Geometry check sheet. Reference: the model listing, model coordinates, mm. A direction names the side the tool comes from. Coordinates: 2 decimals unless noted, no trailing zeros. Loops run counter-clockwise (first coordinate to the right, second up) from the corner with the lowest first, then second, coordinate; pieces in that order, holes last.
from build123d import *

# Parameters (mm, degrees)
F0_W     = 80
F0_H     = 60
F1_DEPTH = 40
F2_W     = 20
F2_H     = 60
F3_DEPTH = 20
F4_W     = 60
F4_H     = 60
F5_DEPTH = 10


with BuildPart() as f1:
    # F0 (on Front) → F1 (new body)
    with BuildSketch(Plane.XZ):
        with Locations((40, 30)):
            Rectangle(F0_W, F0_H)
    extrude(amount=F1_DEPTH)

    # F2 (on face) → F3 (cut)
    with BuildSketch(Plane.XZ.offset(40)):
        with Locations((10, 30)):
            Rectangle(F2_W, F2_H)
        with Locations((70, 30)):
            Rectangle(F2_W, F2_H)
    extrude(amount=-F3_DEPTH, mode=Mode.SUBTRACT)

    # F4 (on face) → F5 (cut)
    with BuildSketch(Plane(origin=(0, 0, 0), x_dir=(-1, 0, 0), z_dir=(0, 1, 0))):
        with Locations((-40, 30)):
            Rectangle(F4_W, F4_H)
    extrude(amount=-F5_DEPTH, mode=Mode.SUBTRACT)


solid = f1.part
(1) Gauge pin test, flat ends, axial feed: pin 1 Ø22 at (x, z) = (74.5, 32) entering from -Y; pin 2 Ø22 at (y, z) = (-33.5, 33) entering from +X; pin 3 Ø1 at (x, z) = (20.5, 33) entering from +Y. Record the tip position at first contact, or that the pin passes through.
Findings:
pin 1: stops at y = -20
pin 2: stops at x = 60
pin 3: stops at y = -10
(2) Sectioned sample at D-D on y = -30. Record the cut outline in (x, z), and give its area (3 significant figures).
Findings:
outline: (20, 0) - (60, 0) - (60, 60) - (20, 60) - close
area: 2,400 mm2
(3) Scan lines: L1, parallel to X at y = -3, z = 54.5; L2, parallel to X at y = -28, z = 14; L3, parallel to Y at x = 22, z = 41.5. Record each from-to range of solid material in increasing order.
Findings:
L1: x = 0 to 10, 70 to 80
L2: x = 20 to 60
L3: y = -40 to -10
(4) Sectioned sample at B-B on z = 40. Record the cut outline in (x, y), and give its area (3 significant figures).
Findings:
outline: (0, -20) - (20, -20) - (20, -40) - (60, -40) - (60, -20) - (80, -20) - (80, 0) - (70, 0) - (70, -10) - (10, -10) - (10, 0) - (0, 0) - close
area: 1,800 mm2
(5) Sectioned sample at C-C on x = 14.5. Record the cut outline in (y, z).
Findings:
outline: (-20, 0) - (-10, 0) - (-10, 60) - (-20, 60) - close
(6) Access from +Z, -Z, +X, -X, +Y, -Y to the whole of each face (thin tool, end or side, straight path). Record for faces 5 (the flat face through (10, -20, 30)), 6 (the flat face through (70, -20, 30)), 7 (the flat face through (70, -5, 30)).
Findings:
face 5: +Z, -Z, -X, -Y
face 6: +Z, -Z, +X, -Y
face 7: +Z, -Z, +Y
(7) Sectioned sample at A-A on y = -7.5. Record the cut outline in (x, z).
Findings:
outline: (0, 0) - (10, 0) - (10, 60) - (0, 60) - close; (70, 0) - (80, 0) - (80, 60) - (70, 60) - close
(8) Draft check along X on faces 1 (the flat face through (20, -30, 30)), 2 (the flat face through (5, 0, 30)), 3 (the flat face through (40, -10, 30)), 4 (the flat face through (10, -5, 30)). Enter one of: +X half, -X half, draft (parallel to the pull), parting line (faces both ways), or undercut.
Findings:
face 1: -X half
face 2: draft
face 3: undercut
face 4: undercut
